```python
from build123d import *

# Parameters (mm, degrees)
EXTRUDE_THIN1_DEPTH = 30
SKETCH2_W           = 30
SKETCH2_H           = 0.984822369
BOSS_EXTRUDE1_DEPTH = 6
SKETCH3_W           = 30
SKETCH3_H           = 0.984822369
BOSS_EXTRUDE2_DEPTH = 6
SKETCH7_W           = 8.024735178
SKETCH7_H           = 30.071065223
BOSS_EXTRUDE3_DEPTH = 7.95
SKETCH9_W           = 8
SKETCH9_H           = 30
BOSS_EXTRUDE5_DEPTH = 7.95


with BuildPart() as part:
    # Sketch1 → Extrude-Thin1 (new body)
    with BuildSketch(Plane.XY):
        with BuildLine():
            ThreePointArc((8, 0), (0, 8), (-8, 0))
            Line((-8, 0), (-10, 0))
            ThreePointArc((-10, 0), (0, 10), (10, 0))
            Line((10, 0), (8, 0))
        make_face()
    extrude(amount=EXTRUDE_THIN1_DEPTH)



with BuildPart() as body_2:
    # Sketch2 → Boss-Extrude1 (new body)
    with BuildSketch(Plane.ZY.offset(10)):
        with Locations((15, 0.492411185)):
            Rectangle(SKETCH2_W, SKETCH2_H)
    extrude(amount=BOSS_EXTRUDE1_DEPTH)


with BuildPart() as body_3:
    # Sketch3 → Boss-Extrude2 (new body)
    with BuildSketch(Plane(origin=(10, 0, 0), x_dir=(0, 0, -1), z_dir=(1, 0, 0))):
        with Locations((-15, 0.492411185)):
            Rectangle(SKETCH3_W, SKETCH3_H)
    extrude(amount=BOSS_EXTRUDE2_DEPTH)


with BuildPart() as part_1:
    add(part.part)

    add(body_3.part)  # Boss-Extrude3 merges body 3
    # Sketch7 → Boss-Extrude3 (add)
    with BuildSketch(Plane(origin=(0, 0, 0), x_dir=(1, 0, 0), z_dir=(0, 1, 0))):
        with Locations((12.012367589, -15.035532612)):
            Rectangle(SKETCH7_W, SKETCH7_H)
    extrude(amount=-BOSS_EXTRUDE3_DEPTH)


    add(body_2.part)  # Boss-Extrude5 merges body 2
    # Sketch9 → Boss-Extrude5 (add)
    with BuildSketch(Plane.XZ):
        with Locations((-12, 15)):
            Rectangle(SKETCH9_W, SKETCH9_H)
    extrude(amount=BOSS_EXTRUDE5_DEPTH)


solid = part_1.part
```
Can you work these out from the model? Positions are in its coordinate system, mm. A direction names the side the tool comes from. Round coordinates to 2 decimals unless told otherwise and drop trailing zeros. Loops run counter-clockwise (first coordinate to the right, second up) from the corner with the lowest first, then second, coordinate; pieces in that order, holes last.
Item 1: Which directions (+Z, -Z, +X, -X, +Y, -Y) give clear straight access to the entire face, cutting with the end or side of a thin tool? Please do faces 1 (the flat face through (-13, 0.985, 15)), 2 (the flat face through (13, 0.5, 30)), 3 (the flat face through (8, -4, 15)), 4 (the flat face through (13, 0.985, 15)).
Item 2: Will these pins go through, and if not, where does the flat tip stop? pin 1 Ø6.5 at (x, z) = (12, 17) entering from +Y; pin 2 Ø0.8 at (y, z) = (0.5, 12) entering from +X; pin 3 Ø10 at (x, y) = (-5.5, -3) entering from +Z; pin 4 Ø5.5 at (x, y) = (-2, 2) entering from +Z.
Item 3: Please list where these lines run through material, in increasing order: L1, parallel to X at y = -3.75, z = 23; L2, parallel to X at y = 5.25, z = 4; L3, parallel to Y at x = 12, z = 15.
Item 4: Suppose I cut it at D-D, the plane x = 0. Write out the boundary of the cut face in (y, z), then the cut area to 3 significant figures.
Item 5: Suppose I cut it at B-B, the plane y = 5.25. Write out the boundary of the cut face in (x, z), then the cut area to 3 significant figures.
Item 6: Suppose I cut it at C-C, the plane x = 11.5. Write out the boundary of the cut face in (y, z).
Reported:
1. face 1: +Z, -Z, -X, +Y
1. face 2: +Z, +X, -X, +Y
1. face 3: +Z, -Z, -Y
1. face 4: +Z, -Z, +X, +Y
2. pin 1: stops at y = 4.84
2. pin 2: stops at x = 16
2. pin 3: stops at z = 30
2. pin 4: passes through
3. L1: x = -16 to -8, 8 to 16.02
3. L2: x = -8.51 to -6.04, 6.04 to 8.51
3. L3: y = -7.95 to 0.98
4. outline: (8, 0) - (10, 0) - (10, 30) - (8, 30) - close
4. area: 60.0 mm2
5. outline: (-8.51, 0) - (-6.04, 0) - (-6.04, 30) - (-8.51, 30) - close; (6.04, 0) - (8.51, 0) - (8.51, 30) - (6.04, 30) - close
5. area: 148 mm2
6. outline: (-7.95, 0) - (0.98, 0) - (0.98, 30) - (0, 30) - (0, 30.07) - (-7.95, 30.07) - close
